Read the model definition and answer for the solid it produces. Units are mm, in the model's axes. Face numbers are marked on the shaded views. A direction names the side the tool comes from. Round coordinates to 2 decimals unless told otherwise and drop trailing zeros. Write each loop counter-clockwise with the first axis right and the second up, starting at its lowest first coordinate (ties: lowest second). Pieces come first, ordered by that corner, then holes. Notation, with made-up numbers: (38, 20) -> (44, 20) arc R22 ccw to (44, 56) -> close; hole circle Ø9 at (-8.5, -21). An arc over 180 degrees is marked (long way). Return JSON: item names as keys, results as strings. Group by question number.
(1) A cutting plane is placed at B-B on x = 0. Give the vertices of the cut face in (y, z), then the cut area to 3 significant figures.
(2) For the marked faces 1 and 2, determine the directions among +Z, -Z, +X, -X, +Y, -Y from which every point of the face is accessible in a straight line to the end or side of a thin tool.
(3) Given pin 1 (1.5 mm diameter, centred on x = -4, z = 19, fed in from -Y); pin 2 (6 mm diameter, centred on y = 4.5, z = 19, fed in from -X); pin 3 (5 mm diameter, centred on x = 0, y = 8, fed in from +Z), each flat-ended and moving along its own axis, determine where each tip first touches the part or whether it passes through.
(4) A cutting plane is placed at A-A on y = 0. Give the vertices of the cut face in (x, z), then the cut area to 3 significant figures.
(5) A cutting plane is placed at C-C on y = -8. Give the vertices of the cut face in (x, z).
(6) A cutting plane is placed at D-D on z = 16.75. Give the vertices of the cut face in (x, y).
(7) Straight lines are drawn through the part: line 1 (Y direction, x = 0, z = 3.05); line 2 (X direction, y = 0.5, z = 4); line 3 (Z direction, x = 2.5, y = -8.25). For each, find the intervals that lie inside material, in ascending order.
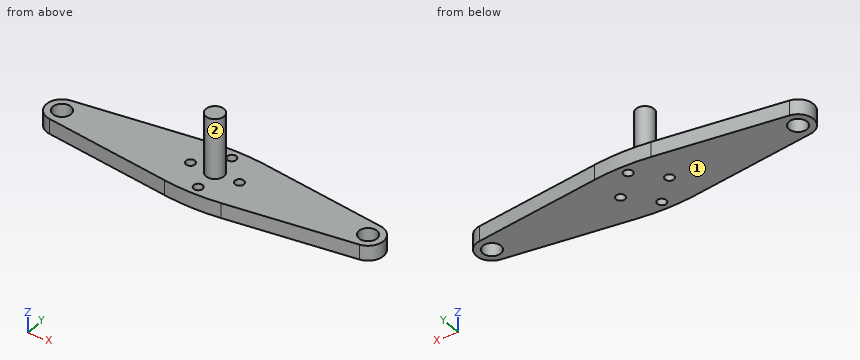
```python
from build123d import *

# Parameters (mm, degrees)
SZKIC1_R                    = 3
SZKIC1_R_2                  = 1.5
DODANIE_WYCI_GNI_CIE1_DEPTH = 5
SZKIC1_2_R                  = 3
DODANIE_WYCI_GNI_CIE2_DEPTH = 25


with BuildPart() as part:
    # Szkic1 → Dodanie-wyci_gni_cie1 (new body)
    with BuildSketch(Plane.XY):
        with BuildLine():
            Line((-50.67287635, 5.055665151), (-9.235111676, 10.570763761))
            ThreePointArc((-9.235111676, 10.570763761), (0, 11.182632843), (9.235111676, 10.570763761))
            Line((9.235111676, 10.570763761), (50.67287635, 5.055665151))
            ThreePointArc((50.67287635, 5.055665151), (55.100246338, 0), (50.67287635, -5.055665151))
            Line((50.67287635, -5.055665151), (9.235111676, -10.570763761))
            ThreePointArc((9.235111676, -10.570763761), (0, -11.182632843), (-9.235111676, -10.570763761))
            Line((-9.235111676, -10.570763761), (-50.67287635, -5.055665151))
            ThreePointArc((-50.67287635, -5.055665151), (-55.100246338, 0), (-50.67287635, 5.055665151))
        make_face()
        Circle(SZKIC1_R, mode=Mode.SUBTRACT)
        with Locations((0, 8)):
            Circle(SZKIC1_R_2, mode=Mode.SUBTRACT)
        with Locations((-8, 0)):
            Circle(SZKIC1_R_2, mode=Mode.SUBTRACT)
        with Locations((8, 0)):
            Circle(SZKIC1_R_2, mode=Mode.SUBTRACT)
        with Locations((0, -8)):
            Circle(SZKIC1_R_2, mode=Mode.SUBTRACT)
        with Locations((-50, 0)):
            Circle(SZKIC1_R, mode=Mode.SUBTRACT)
        with Locations((50, 0)):
            Circle(SZKIC1_R, mode=Mode.SUBTRACT)
    extrude(amount=DODANIE_WYCI_GNI_CIE1_DEPTH)

    # Szkic1_2 → Dodanie-wyci_gni_cie2 (add)
    with BuildSketch(Plane.XY):
        Circle(SZKIC1_2_R)
    extrude(amount=DODANIE_WYCI_GNI_CIE2_DEPTH)


solid = part.part
```
Checks:
{
 "1": {"outline": "(-11.18, 0) -> (-9.5, 0) -> (-9.5, 5) -> (-11.18, 5) -> close; (-6.5, 0) -> (6.5, 0) -> (6.5, 5) -> (3, 5) -> (3, 25) -> (-3, 25) -> (-3, 5) -> (-6.5, 5) -> close; (9.5, 0) -> (11.18, 0) -> (11.18, 5) -> (9.5, 5) -> close", "area": "202 mm^2"},
 "2": {"face 1": "-Z, +X, -X, +Y, -Y", "face 2": "+Z"},
 "3": {"pin 1": "passes through", "pin 2": "stops at x = -2.6", "pin 3": "stops at z = 5"},
 "4": {"outline": "(-55.1, 0) -> (-53, 0) -> (-53, 5) -> (-55.1, 5) -> close; (-47, 0) -> (-9.5, 0) -> (-9.5, 5) -> (-47, 5) -> close; (-6.5, 0) -> (6.5, 0) -> (6.5, 5) -> (3, 5) -> (3, 25) -> (-3, 25) -> (-3, 5) -> (-6.5, 5) -> close; (9.5, 0) -> (47, 0) -> (47, 5) -> (9.5, 5) -> close; (53, 0) -> (55.1, 0) -> (55.1, 5) -> (53, 5) -> close", "area": "581 mm^2"},
 "5": {"outline": "(-28.55, 0) -> (-1.5, 0) -> (-1.5, 5) -> (-28.55, 5) -> close; (1.5, 0) -> (28.55, 0) -> (28.55, 5) -> (1.5, 5) -> close"},
 "6": {"outline": "circle Ø6 at (0, 0)"},
 "7": {"line 1": "y = -11.18 to -9.5, -6.5 to 6.5, 9.5 to 11.18", "line 2": "x = -55.08 to -52.96, -47.04 to -9.41, -6.59 to 6.59, 9.41 to 47.04, 52.96 to 55.08", "line 3": "z = 0 to 5"}
}
